from build123d import *

# Parameters (mm, degrees)
SKIZZE1_W                       = 85
SKIZZE1_H                       = 58.8
AUFSATZ_LINEAR_AUSTRAGEN1_DEPTH = 5
SKIZZE2_W                       = 60
SKIZZE2_H                       = 35
SCHNITT_LINEAR_AUSTRAGEN1_DEPTH = 104.476760676
VERRUNDUNG1_R                   = 10
SKIZZE3_W                       = 15
SKIZZE3_H                       = 5
AUFSATZ_LINEAR_AUSTRAGEN2_DEPTH = 5


with BuildPart() as part:
    # Skizze1 → Aufsatz-Linear austragen1 (new body)
    with BuildSketch(Plane.XY):
        with Locations((42.5, 29.4)):
            Rectangle(SKIZZE1_W, SKIZZE1_H)
    extrude(amount=AUFSATZ_LINEAR_AUSTRAGEN1_DEPTH)

    # Skizze2 → Schnitt-Linear austragen1 (cut, through all)
    with BuildSketch(Plane.XY.offset(5)):
        with Locations((42.5, 32.5)):
            Rectangle(SKIZZE2_W, SKIZZE2_H)
    extrude(amount=-SCHNITT_LINEAR_AUSTRAGEN1_DEPTH, mode=Mode.SUBTRACT)

    # Verrundung1
    verrundung1_edges = [part.edges().sort_by_distance(p)[0] for p in [
        (12.5, 15, 2.5),
        (12.5, 50, 2.5),
        (72.5, 50, 2.5),
        (72.5, 15, 2.5),
    ]]
    fillet(verrundung1_edges, radius=VERRUNDUNG1_R)

    # Skizze3 → Aufsatz-Linear austragen2 (add)
    with BuildSketch(Plane(origin=(0, 58.8, 0), x_dir=(1, 0, 0), z_dir=(0, 1, 0))):
        with Locations((65, -2.5)):
            Rectangle(SKIZZE3_W, SKIZZE3_H)
        with Locations((20, -2.5)):
            Rectangle(SKIZZE3_W, SKIZZE3_H)
    extrude(amount=AUFSATZ_LINEAR_AUSTRAGEN2_DEPTH)


solid = part.part
Work out the finished part from the listing and answer in its coordinate system (mm). A direction names the side the tool comes from. Round coordinates to 2 decimals unless told otherwise and drop trailing zeros. Loops run counter-clockwise (first coordinate to the right, second up) from the corner with the lowest first, then second, coordinate; pieces in that order, holes last. Notation, with made-up numbers: (74.25, 7) - (99.25, 7) arc R34 cw to (99.25, 40) - close; hole circle Ø10 at (57, 61). An arc over 180 degrees is marked (long way). One line per item, written item: value.
Q1. Find section A-A on x = 29.5. Give the vertices of the cut face in (y, z), and give its area (3 significant figures).
Check values:
outline: (0, 0) - (15, 0) - (15, 5) - (0, 5) - close; (50, 0) - (58.8, 0) - (58.8, 5) - (50, 5) - close
area: 119 mm2
Q2. Find section D-D on x = 6. Give the vertices of the cut face in (y, z).
Check values:
outline: (0, 0) - (58.8, 0) - (58.8, 5) - (0, 5) - close
Q3. Each of these flat-tipped pins is pushed along its axis until it touches: pin 1 Ø1.5 at (y, z) = (61.5, 3) entering from -X; pin 2 Ø1.5 at (x, z) = (77.5, 3) entering from +Y; pin 3 Ø1.5 at (y, z) = (62, 1.5) entering from +X. Where does it stop, or does it pass through?
Check values:
pin 1: x = 12.5
pin 2: y = 58.8
pin 3: x = 72.5
Q4. Find section C-C on y = 34. Give the vertices of the cut face in (x, z).
Check values:
outline: (0, 0) - (12.5, 0) - (12.5, 5) - (0, 5) - close; (72.5, 0) - (85, 0) - (85, 5) - (72.5, 5) - close
Q5. Straight lines are drawn through the part: probe 1 along Y at (x, z) = (61, 0.75); probe 2 along Y at (x, z) = (50.5, 3.9); probe 3 along X at (y, z) = (28, 1.6). For each, find the intervals that lie inside material, in ascending order.
Check values:
probe 1: 0 to 15, 50 to 63.8
probe 2: 0 to 15, 50 to 58.8
probe 3: 0 to 12.5, 72.5 to 85
Q6. The mould has two halves that part along Y. Classify faces 1 (the flat face through (20, 63.8, 2)), 2 (the flat face through (12.5, 32, 3)), 3 (the flat face through (0, 29, 2)): +Y half, -Y half, draft (parallel to the pull), parting line (faces both ways), or undercut.
Check values:
face 1: +Y half
face 2: undercut
face 3: draft
Q7. For faces 4 (the flat face through (12.5, 61, 3)), 5 (the cylindrical face through (15.51, 47.15, 2.46)), 6 (the flat face through (57.5, 61, 3)), 7 (the flat face through (79, 58.8, 2)), determine the directions among +Z, -Z, +X, -X, +Y, -Y from which every point of the face is accessible in a straight line to the end or side of a thin tool.
Check values:
face 4: +Z, -Z, -X, +Y
face 5: +Z, -Z
face 6: +Z, -Z, +Y
face 7: +Z, -Z, +X, +Y
Q8. Find section B-B on z = 4.05. Give the vertices of the cut face in (x, y), and give its area (3 significant figures).
Check values:
outline: (0, 0) - (85, 0) - (85, 58.8) - (72.5, 58.8) - (72.5, 63.8) - (57.5, 63.8) - (57.5, 58.8) - (27.5, 58.8) - (27.5, 63.8) - (12.5, 63.8) - (12.5, 58.8) - (0, 58.8) - close; hole (12.5, 25) arc R10 ccw to (22.5, 15) - (62.5, 15) arc R10 ccw to (72.5, 25) - (72.5, 40) arc R10 ccw to (62.5, 50) - (22.5, 50) arc R10 ccw to (12.5, 40) - close
area: 3,130 mm2
